Check sheet for the modelled part. Datum: model origin and axes. Units: mm. Round coordinates to 2 decimals unless told otherwise and drop trailing zeros. Write each loop counter-clockwise with the first axis right and the second up, starting at its lowest first coordinate (ties: lowest second). Pieces come first, ordered by that corner, then holes. Notation, with made-up numbers: M -24,69.25 L 23,69.25 A27 cw 23,90.25 Z; hole C 37,74.25 d6. An arc over 180 degrees is marked long. Put each result on its own line as item: value.
```python
from build123d import *

# Parameters (mm, degrees)
BOX002_W               = 10
BOX002_H               = 16.5
BOX002_DEPTH           = 34
CYLINDER009_R          = 20.75
CYLINDER009_DEPTH      = 150
CYLINDER014_R          = 48
CYLINDER014_DEPTH      = 245
CYLINDER014_ROLL_ANGLE = 90
CYLINDER013_R          = 24
CYLINDER013_DEPTH      = 56


with BuildPart() as obj1:
    # Box002 → Box002 (new body)
    with BuildSketch(Plane(origin=(-32.5, -7.5, -10), x_dir=(1, 0, 0), z_dir=(0, 0, 1))):
        with Locations((5, 8.25)):
            Rectangle(BOX002_W, BOX002_H)
    extrude(amount=BOX002_DEPTH)


with BuildPart() as cylinder009:
    # Cylinder009 → Cylinder009 (new body)
    with BuildSketch(Plane.XY.offset(-32)):
        Circle(CYLINDER009_R)
    extrude(amount=CYLINDER009_DEPTH)


with BuildPart() as cylinder014:
    # Cylinder014 → Cylinder014 (new body)
    with BuildSketch(Plane.XY):
        Circle(CYLINDER014_R)
    extrude(amount=CYLINDER014_DEPTH)


with BuildPart() as cylinder014_1:
    # Cylinder014 roll: moved
    add(cylinder014.part.rotate(Axis((0, 0, 0), (1, 0, 0)), CYLINDER014_ROLL_ANGLE))


with BuildPart() as cylinder014_2:
    # Cylinder014 placement: moved
    add(cylinder014_1.part.moved(Location((0, 79, -47))))


with BuildPart() as fusion009:
    # Cylinder013 → Cylinder013 (new body)
    with BuildSketch(Plane.XY.offset(-32)):
        Circle(CYLINDER013_R)
    extrude(amount=CYLINDER013_DEPTH)

    # Cut008: cut Cylinder014
    add(cylinder014_2.part, mode=Mode.SUBTRACT)

    # Cut009: cut Cylinder009
    add(cylinder009.part, mode=Mode.SUBTRACT)

    # Fusion009: union obj1
    add(obj1.part)


solid = fusion009.part
```
1. Release check for a two-part mould opening along Y. For faces 1 (the flat face through (-28, -7.5, 7)), 2 (the flat face through (-32.5, 1, 7)), 3 (the flat face through (-28, 9, 7)), 4 (the cylindrical face through (19.168, -7.947, 9.948)) record: +Y half, -Y half, draft (parallel to the pull), parting line (faces both ways), or undercut.
Computed values:
face 1: -Y half
face 2: draft
face 3: +Y half
face 4: undercut
2. Cross-section at C-C (z = -2.5). Enter the section's corners in (x, y).
Computed values:
outline: M -32.5,-7.5 L -22.8,-7.5 A24 ccw -17.99,-15.88 L -17.99,-10.34 A20.75 cw -17.99,10.34 L -17.99,15.88 A24 ccw -22.5,8.35 L -22.5,9 L -32.5,9 Z; M 17.99,-15.88 A24 ccw 17.99,15.88 L 17.99,10.34 A20.75 cw 17.99,-10.34 Z
3. Cross-section at B-B (y = 2.5). Enter the section's corners in (x, z).
Computed values:
outline: M -32.5,-10 L -22.5,-10 L -22.5,-4.6 A48 cw -20.6,-3.64 L -20.6,24 L -32.5,24 Z; M 20.6,-3.64 A48 cw 23.87,-5.36 L 23.87,24 L 20.6,24 Z
4. Cross-section at A-A (x = 0). Enter the section's corners in (y, z), then the cut area to 4 significant figures.
Computed values:
outline: M -24,1 L -20.75,1 L -20.75,24 L -24,24 Z; M 20.75,1 L 24,1 L 24,24 L 20.75,24 Z
area: 149.5 mm2
5. Depth check by flat-ended pin: pin 1 Ø8 at (x, z) = (-25.5, 12) entering from +Y; pin 2 Ø12 at (x, z) = (-7, 13) entering from -Y; pin 3 Ø3 at (y, z) = (-15, 12) entering from +X. Enter the tip coordinate at first touch or a pass-through.
Computed values:
pin 1: stops at y = 10.67
pin 2: stops at y = -23.98
pin 3: stops at x = 19.84
6. Scan lines: probe 1 along X at (y, z) = (0, 3.5); probe 2 along Y at (x, z) = (0, 16.5); probe 3 along X at (y, z) = (-15.5, 10). Record each from-to range of solid material in increasing order.
Computed values:
probe 1: x = -32.5 to -20.75, 20.75 to 24
probe 2: y = -24 to -20.75, 20.75 to 24
probe 3: x = -18.32 to -13.8, 13.8 to 18.32
7. Cross-section at D-D (z = 20). Enter the section's corners in (x, y), then the cut area to 3 significant figures.
Computed values:
outline: M -32.5,-7.5 L -22.8,-7.5 A24 ccw long -22.5,8.35 L -22.5,9 L -32.5,9 Z; hole C 0,0 d41.5
area: 605 mm2
